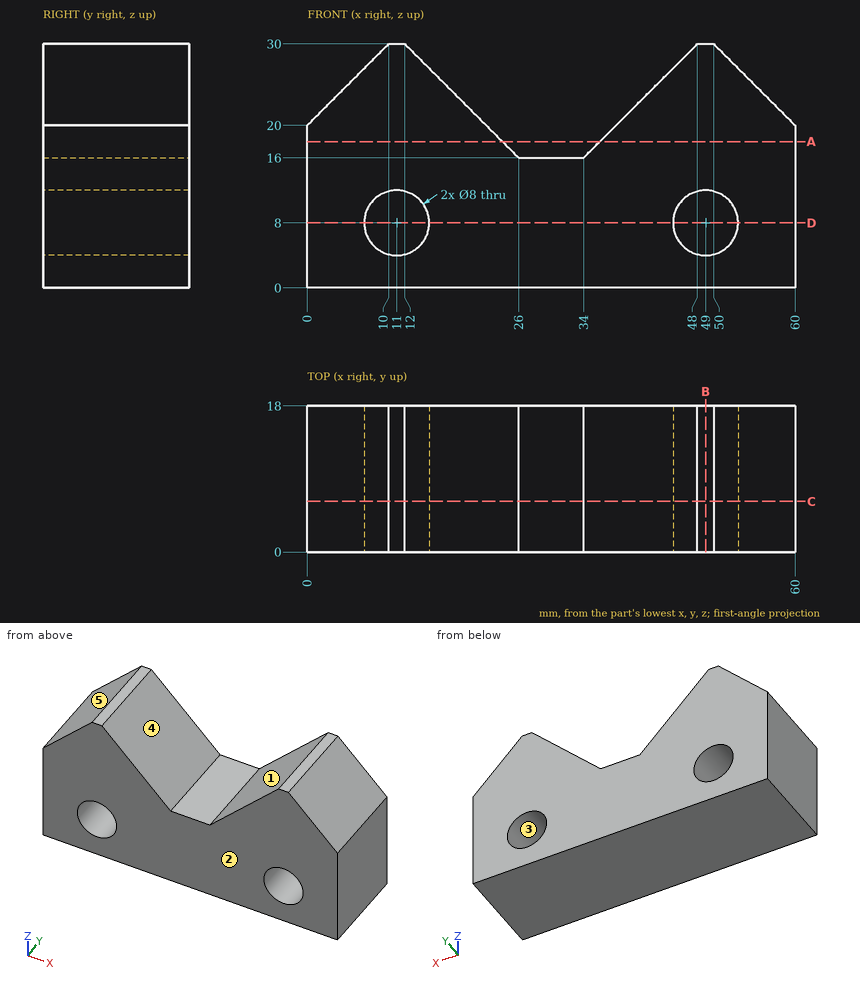
Answer from the drawing. Dimensions are ordinates in mm from the lowest x, y and z of the part. A direction names the side the tool comes from. Coordinates: 2 decimals unless noted, no trailing zeros. Write each loop counter-clockwise with the first axis right and the second up, starting at its lowest first coordinate (ties: lowest second). Pieces come first, ordered by that corner, then holes. Notation, with made-up numbers: (-25.75, 82.5) - (-13.75, 82.5) arc R33 cw to (-13.75, 119.5) - close; hole circle Ø6 at (75.5, 43). An arc over 180 degrees is marked (long way). Return JSON: item names as keys, results as strings. Group by question number.
Q1. For a pull along Z with two mould halves and no side action, classify the marked faces 1, 2 and 3 as +Z half, -Z half, draft (parallel to the pull), parting line (faces both ways), or undercut.
Q2. Find the intervals of material crossed by line 1 along X through (y, z) = (12.25, 8); line 2 along Z through (x, y) = (49, 4.25); line 3 along X through (y, z) = (1.25, 4.5), in increasing order. Write a range as [from, to].
Q3. Which of the six approach directions +Z, -Z, +X, -X, +Y, -Y give full straight-line access (tool end or side, diameter ignored) to the marked faces 4 and 5?
Q4. Flat-ended cylindrical pins translate along their axes: pin 1 Ø5 at (y, z) = (13.5, 21.5) entering from -X; pin 2 Ø9 at (x, y) = (29, 9) entering from +Z; pin 3 Ø1 at (y, z) = (6.5, 21) entering from -X. Find the tip coordinate at first contact, or state that the pin passes through.
Q5. The part is cut by section B-B on x = 49. Write down the section's boundary in (y, z).
Q6. The part is cut by section A-A on z = 18. Write down the section's boundary in (x, y).
Q7. The part is cut by section C-C on y = 6.25. Write down the section's boundary in (x, z).
Q8. The part is cut by section D-D on z = 8. Write down the section's boundary in (x, y).
Evaluation:
{
 "1": {"face 1": "+Z half", "face 2": "draft", "face 3": "undercut"},
 "2": {"line 1": "x = [0, 7], [15, 45], [53, 60]", "line 2": "z = [0, 4], [12, 30]", "line 3": "x = [0, 9.06], [12.94, 47.06], [50.94, 60]"},
 "3": {"face 4": "+Z, +Y, -Y", "face 5": "+Z, -X, +Y, -Y"},
 "4": {"pin 1": "stops at x = 0", "pin 2": "stops at z = 17.5", "pin 3": "stops at x = 0.5"},
 "5": {"outline": "(0, 0) - (18, 0) - (18, 4) - (0, 4) - close; (0, 12) - (18, 12) - (18, 30) - (0, 30) - close"},
 "6": {"outline": "(0, 0) - (24, 0) - (24, 18) - (0, 18) - close; (36, 0) - (60, 0) - (60, 18) - (36, 18) - close"},
 "7": {"outline": "(0, 0) - (60, 0) - (60, 20) - (50, 30) - (48, 30) - (34, 16) - (26, 16) - (12, 30) - (10, 30) - (0, 20) - close; hole circle Ø8 at (11, 8); hole circle Ø8 at (49, 8)"},
 "8": {"outline": "(0, 0) - (7, 0) - (7, 18) - (0, 18) - close; (15, 0) - (45, 0) - (45, 18) - (15, 18) - close; (53, 0) - (60, 0) - (60, 18) - (53, 18) - close"}
}
